Check sheet for the modelled part. Datum: model origin and axes. Units: mm. Coordinates: 2 decimals unless noted, no trailing zeros. Order: outer loops, then holes, each group sorted by start corner. A loop starts at its lowest first (then second) coordinate and runs counter-clockwise, first axis right, second up.
1. Cross-section at A-A (x = 68.58). Enter the section's corners in (y, z) (3 decimals).
2. Cross-section at B-B (x = 44.5). Enter the section's corners in (y, z).
3. Thickness scan on line 1 (Y direction, x = 68.58, z = 1.45) (3 decimals); line 2 (Y direction, x = 68.58, z = 3) (3 decimals); line 3 (Y direction, x = 56, z = 1.7). Record the ranges inside material, lowest first.
4. Gauge pin test, flat ends, axial feed: pin 1 Ø8.5 at (x, y) = (68.58, 60.96) entering from +Z; pin 2 Ø1 at (x, z) = (15, 2) entering from -Y; pin 3 Ø1 at (x, z) = (32, 3) entering from +Y; pin 4 Ø0.6 at (x, y) = (37.5, -73) entering from -Z. Record the tip position at first contact, or that the pin passes through.
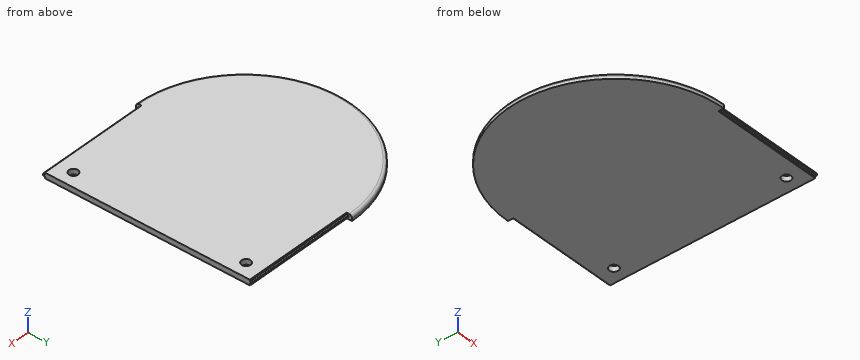
```python
from build123d import *

# Parameters (mm, degrees)
F1_DEPTH = 3.81
F2_W     = 2.54
F2_H     = 3.81
F3_DEPTH = 78.74
F4_W     = 1.27
F4_H     = 1.27
F5_DEPTH = 78.74
F6_R     = 3.175
F7_DEPTH = 25.4
F8_R     = 2.032


# Not quite as in the source:
# - a feature names something its author has since deleted; it is built from what else it names


with BuildPart() as f1:
    # F0 (on Top) → F1 (new body)
    with BuildSketch(Plane.XY):
        with BuildLine():
            Line((0, -76.2), (0, 76.2))
            ThreePointArc((0, 76.2), (-76.2, 0), (0, -76.2))
        make_face()
        with BuildLine():
            ThreePointArc((0, -76.2), (53.8815367264, -53.8815367264), (76.2, 0))
            ThreePointArc((76.2, 0), (53.8815367264, 53.8815367264), (0, 76.2))
            Line((0, 76.2), (0, -76.2))
        make_face()
        with BuildLine():
            ThreePointArc((0, 76.2), (53.8815367264, 53.8815367264), (76.2, 0))
            ThreePointArc((76.2, 0), (53.8815367264, -53.8815367264), (0, -76.2))
            Line((0, -76.2), (78.74, -76.2))
            Line((78.74, -76.2), (78.74, 76.2))
            Line((78.74, 76.2), (0, 76.2))
        make_face()
    extrude(amount=F1_DEPTH)

    # F2 (on face) → F3 (cut)
    with BuildSketch(Plane.YZ.offset(78.74)):
        with Locations((-74.93, 1.905)):
            Rectangle(F2_W, F2_H)
        with Locations((74.93, 1.905)):
            Rectangle(F2_W, F2_H)
    extrude(amount=-F3_DEPTH, mode=Mode.SUBTRACT)

    # F4 (on face) → F5 (cut)
    with BuildSketch(Plane.YZ.offset(78.74)):
        with Locations((-73.025, 3.175)):
            Rectangle(F4_W, F4_H)
        with Locations((-73.025, 0.635)):
            Rectangle(F4_W, F4_H)
        with Locations((73.025, 3.175)):
            Rectangle(F4_W, F4_H)
        with Locations((73.025, 0.635)):
            Rectangle(F4_W, F4_H)
    extrude(amount=-F5_DEPTH, mode=Mode.SUBTRACT)

    # F6 (on face) → F7 (cut)
    with BuildSketch(Plane.XY.offset(3.81)):
        with Locations((68.58, 60.96)):
            Circle(F6_R)
        with Locations((68.58, -60.96)):
            Circle(F6_R)
    extrude(amount=-F7_DEPTH, mode=Mode.SUBTRACT)

    # F8
    f8_edges = [f1.edges().sort_by_distance(p)[0] for p in [
        (-76.2, 0, 3.81),
    ]]
    fillet(f8_edges, radius=F8_R)


solid = f1.part
```
Data:
1. outline: (-73.66, 1.27) - (-72.39, 1.27) - (-72.39, 0) - (-64.135, 0) - (-64.135, 3.81) - (-72.39, 3.81) - (-72.39, 2.54) - (-73.66, 2.54) - close; (-57.785, 0) - (57.785, 0) - (57.785, 3.81) - (-57.785, 3.81) - close; (64.135, 0) - (72.39, 0) - (72.39, 1.27) - (73.66, 1.27) - (73.66, 2.54) - (72.39, 2.54) - (72.39, 3.81) - (64.135, 3.81) - close
2. outline: (-73.66, 1.27) - (-72.39, 1.27) - (-72.39, 0) - (72.39, 0) - (72.39, 1.27) - (73.66, 1.27) - (73.66, 2.54) - (72.39, 2.54) - (72.39, 3.81) - (-72.39, 3.81) - (-72.39, 2.54) - (-73.66, 2.54) - close
3. line 1: y = -73.66 to -64.135, -57.785 to 57.785, 64.135 to 73.66
3. line 2: y = -72.39 to -64.135, -57.785 to 57.785, 64.135 to 72.39
3. line 3: y = -73.66 to 73.66
4. pin 1: stops at z = 3.81
4. pin 2: stops at y = -73.66
4. pin 3: stops at y = 73.66
4. pin 4: stops at z = 1.27
